Source: three-view drawing plus pictorial views. Frame: mm from the lowest corner of the part. Give positions to 0.01 mm unless a question says otherwise; leave off trailing zeros. Order: outer loops, then holes, each group sorted by start corner. A loop starts at its lowest first (then second) coordinate and runs counter-clockwise, first axis right, second up. Notation, with made-up numbers: (-26, -6) -> (33, -6) arc R14 ccw to (33, 8) -> close; hole circle Ø7 at (2, 20.5). An arc over 180 degrees is marked (long way). Use a Markdown table: item, result. Add a question column.
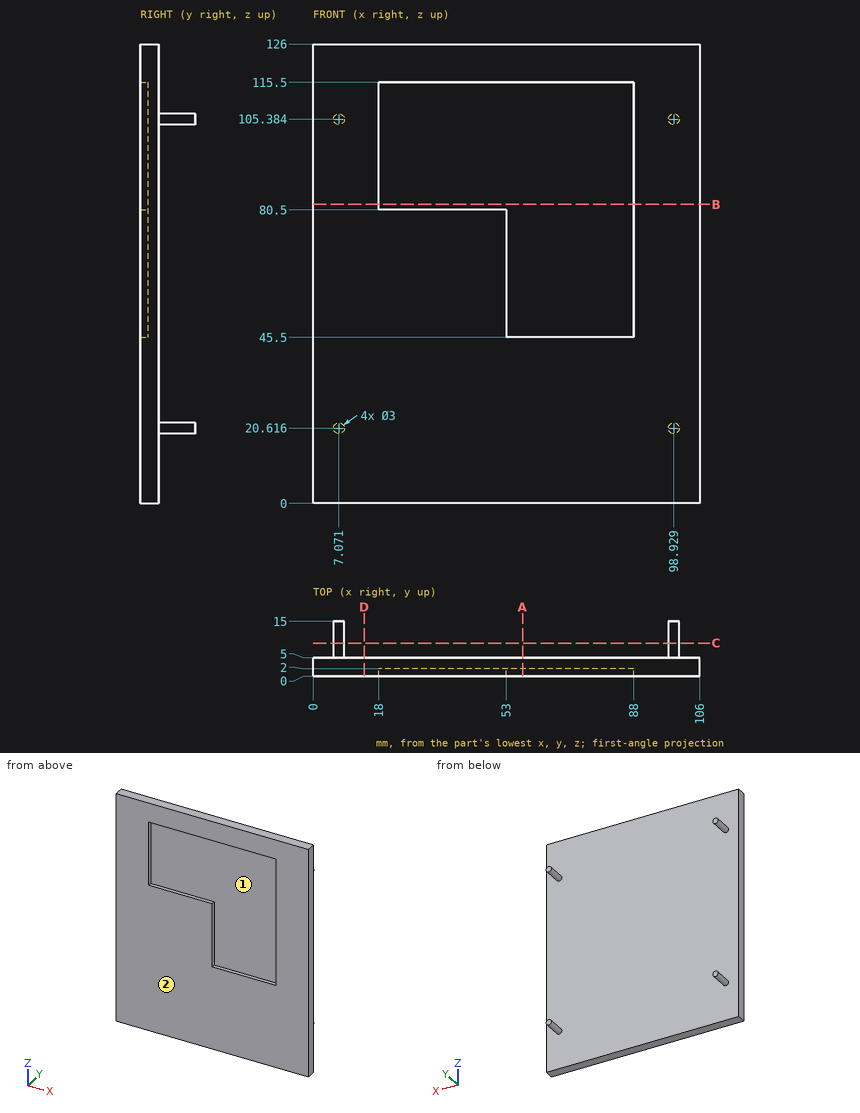
Q1. Section query A-A (x = 57.5). Return loops of the section in (y, z), plus the area to 3 significant figures.
Q2. Section query B-B (z = 82). Return loops of the section in (x, y), plus the area to 3 significant figures.
Q3. Ray query, line 1 (Z direction, x = 7, y = 13.5); line 2 (X direction, y = 6, z = 20.5); line 3 (Y direction, x = 53, z = 100.5). Return the intervals inside material, ascending.
Q4. Section query D-D (x = 14). Return loops of the section in (y, z), plus the area to 3 significant figures.
Q5. Section query C-C (y = 9). Return loops of the section in (x, z), plus the area to 3 significant figures.
Q6. Draft query along Z for the marked faces 1 and 2. Return one class per face: +Z half, -Z half, draft (parallel to the pull), parting line (faces both ways), or undercut.
Q7. First-contact query: pin 1 (2 mm diameter, centred on x = 31.5, z = 37.5, fed in from +Y); pin 2 (3 mm diameter, centred on x = 68, z = 105.5, fed in from -Y). Flat tips, straight axial feed; report the tip coordinate or a pass-through.
Solution:
| question | item | result |
|---|---|---|
| 1 | outline | (0, 0) -> (5, 0) -> (5, 126) -> (0, 126) -> (0, 115.5) -> (2, 115.5) -> (2, 45.5) -> (0, 45.5) -> close |
| 1 | area | 490 mm² |
| 2 | outline | (0, 0) -> (18, 0) -> (18, 2) -> (88, 2) -> (88, 0) -> (106, 0) -> (106, 5) -> (0, 5) -> close |
| 2 | area | 390 mm² |
| 3 | line 1 | z = 19.12 to 22.11, 103.89 to 106.88 |
| 3 | line 2 | x = 5.58 to 8.57, 97.43 to 100.42 |
| 3 | line 3 | y = 2 to 5 |
| 4 | outline | (0, 0) -> (5, 0) -> (5, 126) -> (0, 126) -> close |
| 4 | area | 630 mm² |
| 5 | outline | circle Ø3 at (7.07, 20.62); circle Ø3 at (7.07, 105.38); circle Ø3 at (98.93, 20.62); circle Ø3 at (98.93, 105.38) |
| 5 | area | 28.3 mm² |
| 6 | face 1 | undercut |
| 6 | face 2 | draft |
| 7 | pin 1 | stops at y = 5 |
| 7 | pin 2 | stops at y = 2 |
